Autodesk Inventor part; units mm, degrees
ref_plane "YZ Plane" through (0, 0, 0) normal (1, 0, 0) x (0, 1, 0)
ref_plane "XZ Plane" through (0, 0, 0) normal (0, 1, 0) x (-1, 0, 0)
ref_plane "XY Plane" through (0, 0, 0) normal (0, 0, 1) x (1, 0, 0)
sketch "Sketch1" plane through (0, 0, 0) normal (0, 0, 1) x (1, 0, 0)
  circle A0 centre (0, 0) radius 3.9688
  dimension "d0" = 7.9375
extrude "Extrusion1" add sketch "Sketch1" along normal blind 6.35
sketch "Sketch2" plane through (0, 0, 6.35) normal (0, 0, 1) x (1, 0, 0)
  circle A0 centre (0, 0) radius 3.9688
  circle A1 centre (0, 0) radius 2.413
  dimension "d4" = 4.826
extrude "Extrusion2" add sketch "Sketch2" along normal blind 8.89 contours A1
thread "Thread1"
sketch "Sketch3" plane through (0, 0, 15.24) normal (0, 0, 1) x (1, 0, 0)
  circle A0 centre (0, 0) radius 2.413
  circle A1 centre (0, 0) radius 1.8986
  dimension "d17" = 3.7973
extrude "Extrusion3" add sketch "Sketch3" along normal blind 41.91 contours A1
sketch "Sketch4" plane through (0, 0, 0) normal (0, 0, -1) x (-1, 0, 0)
  circle A0 centre (0, 0) radius 3.9688
  line L0 (-2.2914, 0) -> (-1.1457, 1.9844)
  line L1 (-1.1457, 1.9844) -> (1.1457, 1.9844)
  line L2 (1.1457, 1.9844) -> (2.2914, 0)
  line L3 (2.2914, 0) -> (1.1457, -1.9844)
  line L4 (1.1457, -1.9844) -> (-1.1457, -1.9844)
  line L5 (-1.1457, -1.9844) -> (-2.2914, 0)
  dimension "d23" = 3.9688
extrude "Extrusion4" cut sketch "Sketch4" against normal blind 3.175 contours L0 L1 L2 L3 L4 L5
chamfer "Chamfer1" distance 0.254 angle 45 3 edges at (-3.9688, 0, 0) (-3.9688, 0, 6.35) (-1.8986, 0, 57.15)
chamfer "Chamfer2" distance 0.127 angle 45 1 edges at (-2.413, 0, 15.24)
properties part number "Rod Bolt Side"
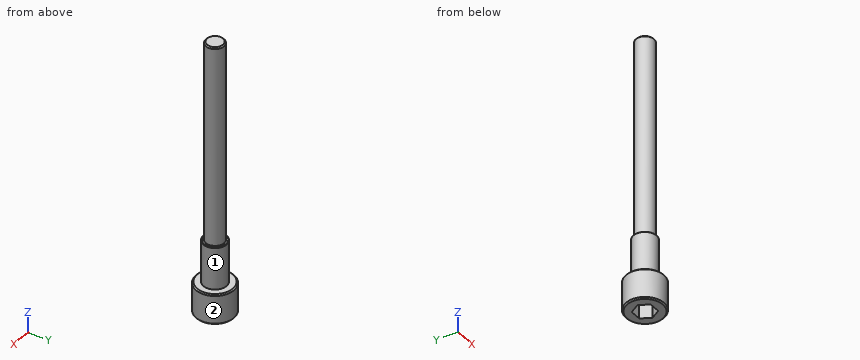
CAD build for the part. Positions are in the model's coordinates, mm. Face numbers are marked on the shaded views. A direction names the side the tool comes from. Give positions to 0.01 mm unless a question says otherwise; leave off trailing zeros. Order: outer loops, then holes, each group sorted by start corner. A loop starts at its lowest first (then second) coordinate and runs counter-clockwise, first axis right, second up. Notation, with made-up numbers: (59.25, 1.5) -> (117.25, 1.5) arc R36 cw to (117.25, 40.5) -> close; hole circle Ø6 at (83, -30). An arc over 180 degrees is marked (long way). Return JSON: item names as keys, results as strings.
Q1. Which spindle directions (+Z, -Z, +X, -X, +Y, -Y) get a long thin tool onto all of the face, cutting with end or side? Do the marked faces 1 and 2. Say none if no direction does.
Working result:
{"face 1": "+Z", "face 2": "+Z, -Z"}
Q2. Drill centre lines: line 1 (Z direction, x = 3.25, y = 1.25); line 2 (Z direction, x = -1, y = 0) (3 decimals); line 3 (Y direction, x = -0.5, z = 38). Where is each one in solid material? Low to high.
Working result:
{"line 1": "0 to 6.35", "line 2": "3.175 to 57.15", "line 3": "-1.83 to 1.83"}
Q3. Saw through at B-B (z = 27). Write the cut outline in (x, y), then the cut area to 3 significant figures.
Working result:
{"outline": "circle Ø3.8 at (0, 0)", "area": "11.3 mm²"}
Q4. Saw through at A-A (x = 0). Write the cut outline in (y, z) (3 decimals), then the cut area to 3 significant figures.
Working result:
{"outline": "(-3.969, 0.254) -> (-3.715, 0) -> (-1.984, 0) -> (-1.984, 3.175) -> (1.984, 3.175) -> (1.984, 0) -> (3.715, 0) -> (3.969, 0.254) -> (3.969, 6.096) -> (3.715, 6.35) -> (2.413, 6.35) -> (2.413, 15.113) -> (2.286, 15.24) -> (1.899, 15.24) -> (1.899, 56.896) -> (1.645, 57.15) -> (-1.645, 57.15) -> (-1.899, 56.896) -> (-1.899, 15.24) -> (-2.286, 15.24) -> (-2.413, 15.113) -> (-2.413, 6.35) -> (-3.715, 6.35) -> (-3.969, 6.096) -> close", "area": "240 mm²"}
Q5. Saw through at C-C (z = 8.5). Write the cut outline in (x, y).
Working result:
{"outline": "circle Ø4.83 at (0, 0)"}
Q6. Flat gauge pins, fed straight in: pin 1 (4 mm diameter, centred on y = -1.5, z = 22.5, fed in from +X); pin 2 (3 mm diameter, centred on x = -1, y = 0.5, fed in from -Z); pin 3 (1.5 mm diameter, centred on y = 2, z = 17.5, fed in from +X). Where does each tip first touch, or does it go through?
Working result:
{"pin 1": "x = 1.9", "pin 2": "z = 0", "pin 3": "x = 1.43"}
